Source: CAD feature listing. Evaluate the final solid. Frame: model axes, mm. A direction names the side the tool comes from. Round coordinates to 2 decimals unless told otherwise and drop trailing zeros. Write each loop counter-clockwise with the first axis right and the second up, starting at its lowest first coordinate (ties: lowest second). Pieces come first, ordered by that corner, then holes. Notation, with made-up numbers: M -32,71.25 L -12,71.25 A14 cw -12,89.25 Z; hole C -24,-36.5 d11. An arc over 180 degrees is marked long. Use a Markdown table: item, result.
```python
from build123d import *

# Parameters (mm, degrees)
F0_W      = 200
F0_H      = 100
F1_DEPTH  = 20
F3_DEPTH  = 10
F5_DEPTH  = 10
F6_R      = 45
F7_DEPTH  = 10
F8_R      = 30
F9_DEPTH  = 32
F11_D     = 10
F11_DEPTH = 15
F11_TIP   = 3.0043030951


# Not quite as in the source:
# - a feature names something its author has since deleted; it is built from what else it names


with BuildPart() as f1:
    # F0 (on Front) → F1 (new body)
    with BuildSketch(Plane.XZ):
        Rectangle(F0_W, F0_H)
    extrude(amount=F1_DEPTH)

    # F2 (on face) → F3 (cut)
    with BuildSketch(Plane.XZ.offset(20)):
        with BuildLine():
            Line((-75, 40), (-81, 40))
            ThreePointArc((-81, 40), (-89.4852813742, 36.4852813742), (-93, 28))
            Line((-93, 28), (-93, -28))
            ThreePointArc((-93, -28), (-89.4852813742, -36.4852813742), (-81, -40))
            Line((-81, -40), (-75, -40))
            ThreePointArc((-75, -40), (-66.5147186258, -36.4852813742), (-63, -28))
            Line((-63, -28), (-63, 28))
            ThreePointArc((-63, 28), (-66.5147186258, 36.4852813742), (-75, 40))
        make_face()
    extrude(amount=-F3_DEPTH, mode=Mode.SUBTRACT)

    # F4 (on face) → F5 (join)
    with BuildSketch(Plane.XZ.offset(20)):
        with BuildLine():
            Line((45.028, 48), (-43, 48))
            ThreePointArc((-43, 48), (-50.0710678119, 45.0710678119), (-53, 38))
            Line((-53, 38), (-53, -38))
            ThreePointArc((-53, -38), (-50.0710678119, -45.0710678119), (-43, -48))
            Line((-43, -48), (45.028, -48))
            ThreePointArc((45.028, -48), (49.6343185527, -47.0344012956), (53.515, -44.3715338615))
            Line((53.515, -44.3715338615), (86.5275302355, -10.4637753147))
            ThreePointArc((86.5275302355, -10.4637753147), (90.7799947329, -0.0125702902), (86.5450528262, 10.4457473475))
            Line((86.5450528262, 10.4457473475), (53.640042261, 44.356597878))
            ThreePointArc((53.640042261, 44.356597878), (49.7035120288, 47.0516780295), (45.028, 48))
        make_face()
    extrude(amount=F5_DEPTH)

    # F6 (on face) → F7 (join)
    with BuildSketch(Plane.XZ.offset(30)):
        Circle(F6_R)
    extrude(amount=F7_DEPTH)

    # F8 (on face) → F9 (cut)
    with BuildSketch(Plane.XZ.offset(40)):
        Circle(F8_R)
    extrude(amount=-F9_DEPTH, mode=Mode.SUBTRACT)

    # F11
    with Locations(Plane.XZ.offset(40)):
        with Locations((-37.5, 0), (0, 37.5), (37.5, 0), (0, -37.5)):
            Hole(F11_D / 2, depth=F11_DEPTH)
            with Locations((0, 0, -(F11_DEPTH + F11_TIP / 2))):  # 118° drill point
                Cone(0, F11_D / 2, F11_TIP, mode=Mode.SUBTRACT)


solid = f1.part
```
Q1. Section B-B on x = 64. Return loops of the section in (y, z).
Results are:
| item | result |
|---|---|
| outline | M -30,-33.6 L -20,-33.6 L -20,-50 L 0,-50 L 0,50 L -20,50 L -20,33.68 L -30,33.68 Z |
Q2. Reachability of faces 4 (the cylindrical face through (49.57, -24.93, -47.06)), 5 (the flat face through (2, -25, 48)), 6 (the flat face through (-78, -10, 1)) from +Z, -Z, +X, -X, +Y, -Y: full face, straight path, thin tool, end or side. Return the list, or none.
Results are:
| item | result |
|---|---|
| face 4 | -Z, +X, -Y |
| face 5 | +Z, +X, -X, -Y |
| face 6 | -Y |
Q3. Section A-A on y = -12. Return loops of the section in (x, z), plus the area to 3 significant figures.
Results are:
| item | result |
|---|---|
| outline | M -100,-50 L 100,-50 L 100,50 L -100,50 Z; hole M -93,-28 A12 ccw -81,-40 L -75,-40 A12 ccw -63,-28 L -63,28 A12 ccw -75,40 L -81,40 A12 ccw -93,28 Z; hole C 0,0 d60 |
| area | 14,900 mm^2 |
Q4. Line query: L1, parallel to Z at x = 0, y = -33; L2, parallel to Z at x = 0, y = -18; L3, parallel to X at y = -14.5, z = 19. Output: solid intervals per line, ascending.
Results are:
| item | result |
|---|---|
| L1 | -45 to -42.5, -32.5 to -30, 30 to 32.5, 42.5 to 45 |
| L2 | -50 to -30, 30 to 50 |
| L3 | -100 to -93, -63 to -23.22, 23.22 to 100 |
Q5. First-contact query: pin 1 Ø12 at (x, z) = (56.5, 13.5) entering from +Y; pin 2 Ø11 at (x, y) = (-12.5, -27.5) entering from -Z; pin 3 Ø8 at (x, z) = (-51.5, -17.5) entering from -Y; pin 4 Ø24 at (x, z) = (-82.5, -8.5) entering from -Y. Flat tips, straight axial feed; report the tip coordinate or a pass-through.
Results are:
| item | result |
|---|---|
| pin 1 | y = 0 |
| pin 2 | z = -48 |
| pin 3 | y = -30 |
| pin 4 | y = -20 |
Q6. Mould query, pull axis X, two halves, no side actions, for faces 1 (the cylindrical face through (-66.42, -15.07, 36.39)), 2 (the flat face through (-0.5, -20, 48.4)), 3 (the cylindrical face through (90.78, -24.93, -0.17)). Classes: +X half, -X half, draft (parallel to the pull), parting line (faces both ways), or undercut.
Results are:
| item | result |
|---|---|
| face 1 | undercut |
| face 2 | draft |
| face 3 | +X half |
